Source: CAD feature listing. Evaluate the final solid. Frame: model axes, mm. A direction names the side the tool comes from. Give positions to 0.01 mm unless a question says otherwise; leave off trailing zeros. Order: outer loops, then holes, each group sorted by start corner. A loop starts at its lowest first (then second) coordinate and runs counter-clockwise, first axis right, second up. Notation, with made-up numbers: (55, 77.25) - (104, 77.25) arc R14 ccw to (104, 104.25) - close; hole circle Ø7 at (66.5, 21). An arc over 180 degrees is marked (long way). Use CSV: the item, a comma, the result in double quotes.
```python
from build123d import *

# Parameters (mm, degrees)
SKETCH1_R           = 5.95
SKETCH1_R_2         = 1.586
BOSS_EXTRUDE1_DEPTH = 7.4
SKETCH2_R           = 3.5
SKETCH2_R_2         = 1.586
BOSS_EXTRUDE2_DEPTH = 7.54
SKETCH3_R           = 1.25
CUT_EXTRUDE1_DEPTH  = 10


with BuildPart() as part:
    # Sketch1 → Boss-Extrude1 (new body)
    with BuildSketch(Plane(origin=(0, 0, 0), x_dir=(1, 0, 0), z_dir=(0, 1, 0))):
        Circle(SKETCH1_R)
        Circle(SKETCH1_R_2, mode=Mode.SUBTRACT)
    extrude(amount=BOSS_EXTRUDE1_DEPTH)

    # Sketch2 → Boss-Extrude2 (add)
    with BuildSketch(Plane.XZ):
        Circle(SKETCH2_R)
        Circle(SKETCH2_R_2, mode=Mode.SUBTRACT)
    extrude(amount=BOSS_EXTRUDE2_DEPTH)

    # Sketch3 → Cut-Extrude1 (cut)
    with BuildSketch(Plane(origin=(0, 0, 0), x_dir=(0, 0, -1), z_dir=(1, 0, 0))):
        with Locations((0, -3.77)):
            Circle(SKETCH3_R)
    extrude(amount=-CUT_EXTRUDE1_DEPTH, mode=Mode.SUBTRACT)


solid = part.part
```
Item 1: Section D-D on x = -2.25. Return the cut outline in (y, z), then the cut area to 3 significant figures.
Filled in:
outline,"(-7.54, -2.68) - (0, -2.68) - (0, -5.51) - (7.4, -5.51) - (7.4, 5.51) - (0, 5.51) - (0, 2.68) - (-7.54, 2.68) - close; hole circle Ø2.5 at (-3.77, 0)"
area,"117 mm2"
Item 2: Set-up query: faces 1 (the cylindrical face through (-2.22, -3.72, 1.25)), 2 (the flat face through (1, -7.54, -2)), 3 (the flat face through (3, 0, 3)). Return all of +Z, -Z, +X, -X, +Y, -Y with unobstructed straight access to the full face (end or side cutting, diameter ignored); none if empty.
Filled in:
face 1,"-X"
face 2,"+Z, -Z, +X, -X, -Y"
face 3,"-Y"
Item 3: Mould query, pull axis X, two halves, no side actions, for faces 4 (the cylindrical face through (1.465, 0.035, -0.607)), 5 (the flat face through (1.24, 7.4, 1.24)), 6 (the cylindrical face through (-4.385, 3.648, -4.021)). Classes: released by +X, released by -X, zero draft, split by the parting line, or undercut.
Filled in:
face 4,"undercut"
face 5,"zero draft"
face 6,"split by the parting line"
Item 4: Material intervals for line 1 (Z direction, x = 0, y = 2.75); line 2 (Y direction, x = -3.5, z = 2.25); line 3 (Z direction, x = -1.55, y = -3.77), sorted ascending. Write a range as from..to.
Filled in:
line 1,"z = -5.95..-1.59, 1.59..5.95"
line 2,"y = 0..7.4"
line 3,"z = -3.14..-1.25, 1.25..3.14"
Item 5: Section B-B on x = 0. Return the cut outline in (y, z), then the cut area to 3 significant figures.
Filled in:
outline,"(-7.54, -3.5) - (0, -3.5) - (0, -5.95) - (7.4, -5.95) - (7.4, -1.59) - (-7.54, -1.59) - close; (-7.54, 1.59) - (7.4, 1.59) - (7.4, 5.95) - (0, 5.95) - (0, 3.5) - (-7.54, 3.5) - close"
area,"93.5 mm2"
Item 6: Section A-A on z = 0. Return the cut outline in (x, y), then the cut area to 3 significant figures.
Filled in:
outline,"(-5.95, 0) - (-3.5, 0) - (-3.5, -2.52) - (-1.59, -2.52) - (-1.59, 7.4) - (-5.95, 7.4) - close; (-3.5, -7.54) - (-1.59, -7.54) - (-1.59, -5.02) - (-3.5, -5.02) - close; (1.59, -7.54) - (3.5, -7.54) - (3.5, 0) - (5.95, 0) - (5.95, 7.4) - (1.59, 7.4) - close"
area,"88.7 mm2"
Item 7: First-contact query: pin 1 (6 mm diameter, centred on y = 0.5, z = -3.5, fed in from +X); pin 2 (4 mm diameter, centred on x = 2.5, y = 1, fed in from -Z); pin 3 (3 mm diameter, centred on y = -4, z = 0.5, fed in from +X). Flat tips, straight axial feed; report the tip coordinate or a pass-through.
Filled in:
pin 1,"stops at x = 5.93"
pin 2,"stops at z = -5.93"
pin 3,"stops at x = 3.5"
Item 8: Section C-C on y = 6.75. Return the cut outline in (x, z), then the cut area to 3 significant figures.
Filled in:
outline,"circle Ø11.9 at (0, 0); hole circle Ø3.17 at (0, 0)"
area,"103 mm2"
